from build123d import *

# Parameters (mm, degrees)
SKETCH_1_W                   = 8
SKETCH_1_H                   = 220
SKETCH_1_R                   = 1.6
EXTRUDE_1_DEPTH              = 3
HOLE_WIZARD_M3_1_D           = 3.4
HOLE_WIZARD_M3_1_DEPTH       = 5
HOLE_WIZARD_M3_1_CSINK_D     = 6.3
HOLE_WIZARD_M3_1_CSINK_ANGLE = 90
HOLE_WIZARD_M3_1_TIP         = 1.021463052
FILLET_1_R                   = 2


with BuildPart() as part:
    # ｽｹｯﾁ1 → ﾎﾞｽ - 押し出し1 (new body)
    with BuildSketch(Plane.XY):
        Rectangle(SKETCH_1_W, SKETCH_1_H)
        with Locations((0, 80)):
            Circle(SKETCH_1_R, mode=Mode.SUBTRACT)
        Circle(SKETCH_1_R, mode=Mode.SUBTRACT)
        with Locations((0, -60)):
            Circle(SKETCH_1_R, mode=Mode.SUBTRACT)
    extrude(amount=EXTRUDE_1_DEPTH)

    # M3 平皿頭ねじ用皿穴1
    with Locations(Plane.XY.offset(3)):
        with Locations((0, -60), (0, 0), (0, 80)):
            CounterSinkHole(HOLE_WIZARD_M3_1_D / 2, HOLE_WIZARD_M3_1_CSINK_D / 2, depth=HOLE_WIZARD_M3_1_DEPTH, counter_sink_angle=HOLE_WIZARD_M3_1_CSINK_ANGLE)
            with Locations((0, 0, -(HOLE_WIZARD_M3_1_DEPTH + HOLE_WIZARD_M3_1_TIP / 2))):  # 118° drill point
                Cone(0, HOLE_WIZARD_M3_1_D / 2, HOLE_WIZARD_M3_1_TIP, mode=Mode.SUBTRACT)

    # ﾌｨﾚｯﾄ1
    # the kernel refuses this fillet: 2 mm, written as the material it takes off along each edge
    with BuildSketch(Plane(origin=(4, 115, 3), x_dir=(-1, 0, 0), z_dir=(0, -1, 0)), Plane(origin=(-4, -115, 3), x_dir=(1, 0, 0), z_dir=(0, 1, 0))) as fillet_1_piece_1:
        with BuildLine():
            CenterArc((FILLET_1_R, FILLET_1_R), FILLET_1_R, 180, 90)
            Line((0, FILLET_1_R), (0, 0))
            Line((0, 0), (FILLET_1_R, 0))
        make_face()
    extrude(amount=230, mode=Mode.SUBTRACT)
    with BuildSketch(Plane(origin=(-9, 110, 3), x_dir=(0, -1, 0), z_dir=(1, 0, 0))) as fillet_1_piece_2:
        with BuildLine():
            CenterArc((FILLET_1_R, FILLET_1_R), FILLET_1_R, 180, 90)
            Line((0, FILLET_1_R), (0, 0))
            Line((0, 0), (FILLET_1_R, 0))
        make_face()
    extrude(amount=18, mode=Mode.SUBTRACT)
    with BuildSketch(Plane(origin=(9, -110, 3), x_dir=(0, 0, -1), z_dir=(-1, 0, 0))) as fillet_1_piece_3:
        with BuildLine():
            CenterArc((FILLET_1_R, -FILLET_1_R), FILLET_1_R, 90, 90)
            Line((0, -FILLET_1_R), (0, 0))
            Line((0, 0), (FILLET_1_R, 0))
        make_face()
    extrude(amount=18, mode=Mode.SUBTRACT)


solid = part.part
Model file for the job. Use its own axes, mm. Give positions to 0.01 mm unless a question says otherwise; leave off trailing zeros. Write each loop counter-clockwise with the first axis right and the second up, starting at its lowest first coordinate (ties: lowest second). Pieces come first, ordered by that corner, then holes. Notation, with made-up numbers: M 78.25,85 L 88.25,85 A24 ccw 88.25,105 Z; hole C 81,62 d1. An arc over 180 degrees is marked long. One line per item, written item: value. Start each with the question number.
Q1. Two-plate mould, pull along Y, no slides. Class faces 1 (the cylindrical face through (0.221, -58.314, 0.764)), 2 (the flat face through (0, -85, 3)): +Y half, -Y half, draft (parallel to the pull), parting line (faces both ways), or undercut.
Q2. Drop flat-ended pins along their axis: pin 1 Ø1 at (x, z) = (-1, 2) entering from -Y; pin 2 Ø2 at (x, y) = (0, 80) entering from +Z. Give the stop position or say it passes through.
Q3. Saw through at B-B, the plane z = 2.05. Write the cut outline in (x, y), plus the area to 3 significant figures.
Q4. Probe probe 1 along Y at (x, z) = (0, 0.45); probe 2 along X at (y, z) = (0, 0.7); probe 3 along Y at (x, z) = (-1.5, 1.45). List the from-to ranges inside material, lowest first. Write a range as [from, to].
Q5. Saw through at A-A, the plane x = 0. Write the cut outline in (y, z), plus the area to 3 significant figures.
Q6. Saw through at C-C, the plane y = -5.5. Write the cut outline in (x, z), plus the area to 3 significant figures.
Output values:
1. face 1: undercut
1. face 2: draft
2. pin 1: stops at y = -109.94
2. pin 2: passes through
3. outline: M -3.7,-109.7 L 3.7,-109.7 L 3.7,109.7 L -3.7,109.7 Z; hole C 0,-60 d4.4; hole C 0,0 d4.4; hole C 0,80 d4.4
3. area: 1,580 mm²
4. probe 1: y = [-110, -61.7], [-58.3, -1.7], [1.7, 78.3], [81.7, 110]
4. probe 2: x = [-4, -1.7], [1.7, 4]
4. probe 3: y = [-109.95, -60.8], [-59.2, -0.8], [0.8, 79.2], [80.8, 109.95]
5. outline: M -110,0 L -61.7,0 L -61.7,1.55 L -63.15,3 L -108,3 A2 ccw -110,1 Z; M -58.3,0 L -1.7,0 L -1.7,1.55 L -3.15,3 L -56.85,3 L -58.3,1.55 Z; M 1.7,0 L 78.3,0 L 78.3,1.55 L 76.85,3 L 3.15,3 L 1.7,1.55 Z; M 81.7,0 L 110,0 L 110,1 A2 ccw 108,3 L 83.15,3 L 81.7,1.55 Z
5. area: 621 mm²
6. outline: M -4,0 L 4,0 L 4,1 A2 ccw 2,3 L -2,3 A2 ccw -4,1 Z
6. area: 22.3 mm²
